```python
from build123d import *

# Parameters (mm, degrees)
VYSUNOUT_TENKOST_NN_1_DEPTH = 600
ODEBRAT_VYSUNUT_M1_DEPTH    = 130


with BuildPart() as part:
    # Skica1 → Vysunout tenkostěnný1 (new body)
    with BuildSketch(Plane(origin=(0, 0, 0), x_dir=(1, 0, 0), z_dir=(0, 1, 0))):
        with BuildLine():
            Line((22.5, -55), (22.5, -62))
            ThreePointArc((22.5, -62), (21.621320344, -64.121320344), (19.5, -65))
            Line((19.5, -65), (-4.5, -65))
            ThreePointArc((-4.5, -65), (-6.621320344, -64.121320344), (-7.5, -62))
            Line((-7.5, -62), (-7.5, -31))
            ThreePointArc((-7.5, -31), (-7.792893219, -30.292893219), (-8.5, -30))
            Line((-8.5, -30), (-19.5, -30))
            ThreePointArc((-19.5, -30), (-21.621320344, -29.121320344), (-22.5, -27))
            Line((-22.5, -27), (-22.5, 62))
            ThreePointArc((-22.5, 62), (-21.621320344, 64.121320344), (-19.5, 65))
            Line((-19.5, 65), (19.5, 65))
            ThreePointArc((19.5, 65), (21.621320344, 64.121320344), (22.5, 62))
            Line((22.5, 62), (22.5, 55))
            Line((22.5, 55), (20.5, 55))
            Line((20.5, 55), (20.5, 62))
            ThreePointArc((20.5, 62), (20.207106781, 62.707106781), (19.5, 63))
            Line((19.5, 63), (-19.5, 63))
            ThreePointArc((-19.5, 63), (-20.207106781, 62.707106781), (-20.5, 62))
            Line((-20.5, 62), (-20.5, -27))
            ThreePointArc((-20.5, -27), (-20.207106781, -27.707106781), (-19.5, -28))
            Line((-19.5, -28), (-8.5, -28))
            ThreePointArc((-8.5, -28), (-6.378679656, -28.878679656), (-5.5, -31))
            Line((-5.5, -31), (-5.5, -62))
            ThreePointArc((-5.5, -62), (-5.207106781, -62.707106781), (-4.5, -63))
            Line((-4.5, -63), (19.5, -63))
            ThreePointArc((19.5, -63), (20.207106781, -62.707106781), (20.5, -62))
            Line((20.5, -62), (20.5, -55))
            Line((20.5, -55), (22.5, -55))
        make_face()
    extrude(amount=VYSUNOUT_TENKOST_NN_1_DEPTH)

    # Skica2 → Odebrat vysunutím1 (cut)
    with BuildSketch(Plane.XY.offset(65)):
        Polygon((22.5, 600), (-22.5, 600), (-22.5, 555), align=None)
    extrude(amount=-ODEBRAT_VYSUNUT_M1_DEPTH, mode=Mode.SUBTRACT)


solid = part.part
```
Input: part model. Units: mm. Frame: model coordinates. A direction names the side the tool comes from. Give positions to 0.01 mm unless a question says otherwise; leave off trailing zeros. Loops run counter-clockwise (first coordinate to the right, second up) from the corner with the lowest first, then second, coordinate; pieces in that order, holes last. Notation, with made-up numbers: M 30,-26.5 L 35,-26.5 A8 cw 35,-11.5 Z; hole C 1,75.25 d11. An arc over 180 degrees is marked long. Answer as CSV lines item,"result". Start each with the question number.
1. Section B-B on y = 370. Return loops of the section in (x, z), plus the area to 3 significant figures.
2. Pull-direction query (Z, two-part tool) for faces 6 (the face through (-21.8, 555.7, 9.9)), 7 (the face through (8, 294, 65)), 8 (the face through (-20.5, 275, -18)); classes: released by +Z, released by -Z, zero draft, split by the parting line, or undercut.
3. Pin query (flat end, axial travel): P1, Ø5.5, axis at y = 238, z = 59, coming from the -X side; P2, Ø1.5, axis at y = 275, z = 35.5, coming from the +X side; P3, Ø1.6, axis at x = 21.5, y = 218.5, coming from the +Z side. Return the tip coordinate at first contact, or that it passes through.
4. Line query: L1, parallel to X at y = 111, z = -57.5; L2, parallel to Z at x = -2, y = 82; L3, parallel to X at y = 442.5, z = 60. Output: solid intervals per line, ascending.
5. Section A-A on x = 3.5. Return loops of the section in (y, z), plus the area to 3 significant figures.
6. Section C-C on z = -44. Return loops of the section in (x, y).
7. Reachability of faces 1 (the face through (-14, 281, 28)), 2 (the face through (7, 294, 63)), 3 (the face through (-22, 0, 5)), 4 (the face through (0, 294, -65)), 5 (the face through (-14, 281, 30)) from +Z, -Z, +X, -X, +Y, -Y: full face, straight path, thin tool, end or side. Return the list, or none.
Computed values:
1,outline,"M -22.5,-62 A3 ccw -19.5,-65 L 19.5,-65 A3 ccw 22.5,-62 L 22.5,-55 L 20.5,-55 L 20.5,-62 A1 cw 19.5,-63 L -19.5,-63 A1 cw -20.5,-62 L -20.5,27 A1 cw -19.5,28 L -8.5,28 A3 ccw -5.5,31 L -5.5,62 A1 cw -4.5,63 L 19.5,63 A1 cw 20.5,62 L 20.5,55 L 22.5,55 L 22.5,62 A3 ccw 19.5,65 L -4.5,65 A3 ccw -7.5,62 L -7.5,31 A1 cw -8.5,30 L -19.5,30 A3 ccw -22.5,27 Z"
1,area,"454 mm²"
2,face 6,"zero draft"
2,face 7,"released by +Z"
2,face 8,"undercut"
3,P1,"stops at x = -7.5"
3,P2,"stops at x = -5.5"
3,P3,"stops at z = 64.75"
4,L1,"x = -22.5 to -20.5, 20.5 to 22.5"
4,L2,"z = -65 to -63, 63 to 65"
4,L3,"x = -7.5 to -5.5, 20.5 to 22.5"
5,outline,"M 0,-65 L 581,-65 L 581,-63 L 0,-63 Z; M 0,63 L 581,63 L 581,65 L 0,65 Z"
5,area,"2,320 mm²"
6,outline,"M -22.5,0 L -20.5,0 L -20.5,557 L -22.5,555 Z"
7,face 1,"+X, +Y, -Y"
7,face 2,"+Y, -Y"
7,face 3,"+Z, -Z, +X, -X, -Y"
7,face 4,"-Z, +X, -X, +Y, -Y"
7,face 5,"+Z, -X, +Y, -Y"
